Part model, mm, in its own coordinate system. A direction names the side the tool comes from. Coordinates: 2 decimals unless noted, no trailing zeros. Loops run counter-clockwise (first coordinate to the right, second up) from the corner with the lowest first, then second, coordinate; pieces in that order, holes last. Notation, with made-up numbers: M 29.25,58 L 48.25,58 A14 cw 48.25,62 Z; hole C 17.5,73 d9. An arc over 180 degrees is marked long. Use a Markdown table: item, result. Add a question column.
1) Pin check, flat tips, straight feed: pin 1 Ø2 at (x, z) = (2.5, -1) entering from -Y; pin 2 Ø3 at (y, z) = (2, 0.5) entering from -X; pin 3 Ø1 at (x, z) = (2.5, 1) entering from +Y; pin 4 Ø2 at (x, y) = (3.5, -1.5) entering from -Z. Stop position of each tip, or through.
2) Band-saw the part on A-A (x = 4.5). List the corners of the cut face in (y, z), plus the area to 3 significant figures.
3) Pull direction Y, two halves, no side cores. Call faces 1 (the cylindrical face through (0.203, 2.685, -0.596)), 2 (the flat face through (0, 1, -1)), 3 (the flat face through (0.943, -1.105, 0.005)): released by +Y, released by -Y, zero draft, split by the parting line, or undercut.
4) Wall check: probe 1 along X at (y, z) = (1.6, -0.4); probe 2 along Z at (x, y) = (0.5, -1.05); probe 3 along X at (y, z) = (-0.05, 2.1). Give the ranges that are in metal, low to high. Write a range as from..to.
5) Tool access for faces 4 (the cylindrical face through (3.917, -1.487, -0.195)), 5 (the flat face through (6, 0, 0)), 6 (the flat face through (0.943, -0.005, -1.105)): list every direction of +Z, -Z, +X, -X, +Y, -Y with a clear straight run to the whole face (end or side of a thin tool).
from build123d import *

# Parameters (mm, degrees)
FILLET1_R    = 0.3
RECPAT_COUNT = 2
RECPAT_ANGLE = 90


with BuildPart() as part:
    # BodySke → BaseBody (revolve)
    with BuildSketch(Plane.XY, mode=Mode.PRIVATE) as basebody_sk:
        Polygon((0, 0), (0, 2.75), (0.4, 2.75), (1.65, 1.5), (6, 1.5), (6, 0), align=None)
    revolve(basebody_sk.sketch.rotate(Axis((0, 0, 0), (1, 0, 0)), 90), axis=Axis((0, 0, 0), (1, 0, 0)))

    # Fillet1
    fillet1_edges = [part.edges().sort_by_distance(p)[0] for p in [
        (1.65, 0, -1.5),
    ]]
    fillet(fillet1_edges, radius=FILLET1_R)

    # RecSkeTop → Recess section 0
    with BuildSketch(Plane.ZY):
        with BuildLine():
            Line((-0.3465, 1.575), (0.3465, 1.575))
            Line((0.3465, 1.575), (0.3465, -1.575))
            Line((0.3465, -1.575), (-0.3465, -1.575))
            Line((-0.3465, -1.575), (-0.3465, 1.575))
        make_face()
    # RecSkeBot → Recess section 1
    with BuildSketch(Plane(origin=(1.86, 0, 0), x_dir=(0, 0, -1), z_dir=(1, 0, 0))):
        with BuildLine():
            Line((0.3465, 0.647638364), (-0.3465, 0.647638364))
            Line((-0.3465, 0.647638364), (-0.3465, -0.647638364))
            Line((-0.3465, -0.647638364), (0.3465, -0.647638364))
            Line((0.3465, -0.647638364), (0.3465, 0.647638364))
        make_face()
    recess = loft(mode=Mode.SUBTRACT)

    # RecPat: Recess ×2 about axis
    recpat_axis = Axis((0, 0, 0), (1, 0, 0))
    for i in range(1, RECPAT_COUNT):
        add(recess.rotate(recpat_axis, i * RECPAT_ANGLE / (RECPAT_COUNT - 1)), mode=Mode.SUBTRACT)

    # RecCorSke → RecessCore (revolve, cut)
    with BuildSketch(Plane.XY, mode=Mode.PRIVATE) as recesscore_sk:
        Polygon((0, 0), (0, 0.7623), (1.86, 0.63223613), (2.065425971, 0), align=None)
    revolve(recesscore_sk.sketch.rotate(Axis((0, 0, 0), (1, 0, 0)), 90), axis=Axis((0, 0, 0), (1, 0, 0)), mode=Mode.SUBTRACT)


solid = part.part
Entries:
| question | item | result |
|---|---|---|
| 1 | pin 1 | y = -1.5 |
| 1 | pin 2 | x = 0 |
| 1 | pin 3 | y = 1.41 |
| 1 | pin 4 | z = -1.41 |
| 2 | outline | C 0,0 d3 |
| 2 | area | 7.07 mm2 |
| 3 | face 1 | split by the parting line |
| 3 | face 2 | zero draft |
| 3 | face 3 | undercut |
| 4 | probe 1 | 0..1.5 |
| 4 | probe 2 | -2.43..-0.35, 0.35..2.43 |
| 4 | probe 3 | 0..1.05 |
| 5 | face 4 | +X |
| 5 | face 5 | +Z, -Z, +X, +Y, -Y |
| 5 | face 6 | -X |
